Read the model definition and answer for the solid it produces. Units are mm, in the model's axes. A direction names the side the tool comes from. Coordinates: 2 decimals unless noted, no trailing zeros. Loops run counter-clockwise (first coordinate to the right, second up) from the corner with the lowest first, then second, coordinate; pieces in that order, holes last. Notation, with made-up numbers: (83, 81) -> (87, 81) arc R26 cw to (87, 101) -> close; hole circle Ø7 at (22.5, 89.25). An arc over 180 degrees is marked (long way). Answer in a Markdown table with one row per item.
```python
from build123d import *

# Parameters (mm, degrees)
EXTRUDE_2_DEPTH     = 2
SKETCH_3_R          = 1.5
CUT_EXTRUDE_1_DEPTH = 95.361008897
EXTRUDE_3_DEPTH     = 1
DRAFT_4_ANGLE       = 43
SKETCH_6_W          = 6
SKETCH_6_H          = 10
EXTRUDE_4_DEPTH     = 5
SKETCH_7_W          = 6
SKETCH_7_H          = 10
EXTRUDE_5_DEPTH     = 5


with BuildPart() as part:
    # 草图1 → 凸台-拉伸2 (new body)
    with BuildSketch(Plane.XY):
        Polygon((0, 0), (0, 50), (20, 50), (20, 40), (60, 40), (60, 50), (80, 50), (80, 0), (60, 0), (60, 10), (20, 10), (20, 0), align=None)
    extrude(amount=EXTRUDE_2_DEPTH)

    # 草图3 → 切除-拉伸1 (cut, through all)
    with BuildSketch(Plane.XY.offset(2)):
        with Locations((10, 45)):
            Circle(SKETCH_3_R)
        with Locations((10, 5)):
            Circle(SKETCH_3_R)
        with Locations((70, 45)):
            Circle(SKETCH_3_R)
        with Locations((70, 5)):
            Circle(SKETCH_3_R)
    extrude(amount=-CUT_EXTRUDE_1_DEPTH, mode=Mode.SUBTRACT)

    # 草图5 → 凸台-拉伸3 (add)
    with BuildSketch(Plane.XY.offset(2)):
        with BuildLine():
            Line((0, 50), (6, 50))
            Line((6, 50), (6, 45))
            ThreePointArc((6, 45), (10, 41), (14, 45))
            Line((14, 45), (14, 50))
            Line((14, 50), (20, 50))
            Line((20, 50), (20, 40))
            Line((20, 40), (60, 40))
            Line((60, 40), (60, 50))
            Line((60, 50), (66, 50))
            Line((66, 50), (66, 45))
            ThreePointArc((66, 45), (70, 41), (74, 45))
            Line((74, 45), (74, 50))
            Line((74, 50), (80, 50))
            Line((80, 50), (80, 0))
            Line((80, 0), (74, 0))
            Line((74, 0), (74, 5))
            ThreePointArc((74, 5), (70, 9), (66, 5))
            Line((66, 5), (66, 0))
            Line((66, 0), (60, 0))
            Line((60, 0), (60, 10))
            Line((60, 10), (20, 10))
            Line((20, 10), (20, 0))
            Line((20, 0), (14, 0))
            Line((14, 0), (14, 5))
            ThreePointArc((14, 5), (10, 9), (6, 5))
            Line((6, 5), (6, 0))
            Line((6, 0), (0, 0))
            Line((0, 0), (0, 50))
        make_face()
    extrude(amount=EXTRUDE_3_DEPTH)

    # 拔模4
    draft_4_faces = [part.faces().sort_by_distance(p)[0] for p in [
        (40, 25, 3),
    ]]
    draft(draft_4_faces, Plane(origin=(20, 0, 2), x_dir=(-1, 0, 0), z_dir=(0, -1, 0)), DRAFT_4_ANGLE)

    # 草图6 → 凸台-拉伸4 (add)
    with BuildSketch(Plane(origin=(0, -1.496346075, 1.604634711), x_dir=(1, 0, 0), z_dir=(0, -0.6819983600624997, 0.7313537016191695))):
        with Locations((3, 7.04599508)):
            Rectangle(SKETCH_6_W, SKETCH_6_H)
    extrude(amount=EXTRUDE_4_DEPTH)

    # 草图7 → 凸台-拉伸5 (add)
    with BuildSketch(Plane(origin=(0, -1.496346075, 1.604634711), x_dir=(1, 0, 0), z_dir=(0, -0.6819983600624997, 0.7313537016191695))):
        with Locations((77, 7.04599508)):
            Rectangle(SKETCH_7_W, SKETCH_7_H)
    extrude(amount=EXTRUDE_5_DEPTH)


solid = part.part
```
1. A cutting plane is placed at B-B on z = 25.5. Give the vertices of the cut face in (x, y).
A:
| item | result |
|---|---|
| outline | (0, 24.13) -> (80, 24.13) -> (80, 50) -> (74, 50) -> (74, 45) arc R4 cw to (66, 45) -> (66, 50) -> (60, 50) -> (60, 40) -> (20, 40) -> (20, 50) -> (14, 50) -> (14, 45) arc R4 cw to (6, 45) -> (6, 50) -> (0, 50) -> close |
2. The mould has two halves that part along Y. Classify faces 4 (the cylindrical face through (9.675, 43.536, 1.014)), 5 (the flat face through (10, 47, 2)), 6 (the flat face through (2.958, 0.298, 10.115)): pulls with the +Y half, pulls with the -Y half, needs draft (parallel to the pull), parting line crosses it, or undercut.
A:
| item | result |
|---|---|
| face 4 | undercut |
| face 5 | needs draft |
| face 6 | pulls with the -Y half |
3. A tool of negligible diameter and unlimited length cuts with its end or side. For faces 1 (the flat face through (76.958, 5.632, 11.623)), 2 (the flat face through (70, 47, 2)), 3 (the flat face through (6, 2, 7)), from which of +Z, -Z, +X, -X, +Y, -Y can it reach the whole face along a straight path? Write none if from no direction.
A:
| item | result |
|---|---|
| face 1 | +Z, +X, -X |
| face 2 | +Z, +Y |
| face 3 | +Z, -Y |
4. Find the intervals of material crossed by probe 1 along Y at (x, z) = (70, 0.95); probe 2 along Y at (x, z) = (58.5, 4); probe 3 along X at (y, z) = (42.5, 41), in increasing order.
A:
| item | result |
|---|---|
| probe 1 | y = 0 to 3.5, 6.5 to 43.5, 46.5 to 50 |
| probe 2 | y = 10 to 40 |
| probe 3 | x = 0 to 6.88, 13.12 to 20, 60 to 66.88, 73.12 to 80 |
5. Given pin 1 Ø10 at (x, z) = (40.5, 5) entering from -Y; pin 2 Ø4 at (x, y) = (11, 43.5) entering from +Z; pin 3 Ø20 at (x, z) = (45, 18) entering from +Y; pin 4 Ø1.8 at (x, y) = (70, 5) entering from -Z, each flat-ended and moving along its own axis, determine where each tip first touches the part or whether it passes through.
A:
| item | result |
|---|---|
| pin 1 | stops at y = 10 |
| pin 2 | stops at z = 2 |
| pin 3 | stops at y = 40 |
| pin 4 | passes through |
6. A cutting plane is placed at A-A on x = 70. Give the vertices of the cut face in (y, z), and give its area (3 significant figures).
A:
| item | result |
|---|---|
| outline | (0, 0) -> (3.5, 0) -> (3.5, 2) -> (0, 2) -> close; (6.5, 0) -> (43.5, 0) -> (43.5, 2) -> (41, 2) -> (41, 41.23) -> (9, 11.39) -> (9, 2) -> (6.5, 2) -> close; (46.5, 0) -> (50, 0) -> (50, 2) -> (46.5, 2) -> close |
| area | 866 mm2 |
7. A cutting plane is placed at C-C on x = 57.5. Give the vertices of the cut face in (y, z), and give its area (3 significant figures).
A:
| item | result |
|---|---|
| outline | (10, 0) -> (40, 0) -> (40, 40.3) -> (10, 12.33) -> close |
| area | 789 mm2 |
8. A cutting plane is placed at D-D on y = 17.5. Give the vertices of the cut face in (x, z), and give its area (3 significant figures).
A:
| item | result |
|---|---|
| outline | (0, 0) -> (80, 0) -> (80, 19.32) -> (0, 19.32) -> close |
| area | 1,550 mm2 |
